CAD build for the part. Positions are in the model's coordinates, mm. A direction names the side the tool comes from. Give positions to 0.01 mm unless a question says otherwise; leave off trailing zeros. Loops run counter-clockwise (first coordinate to the right, second up) from the corner with the lowest first, then second, coordinate; pieces in that order, holes last. Notation, with made-up numbers: M -15,-18.75 L 43,-18.75 A10 cw 43,-0.75 Z; hole C -25.75,65.25 d2. An arc over 180 degrees is marked long. Answer as CSV lines item,"result".
from build123d import *

# Parameters (mm, degrees)
BOSS_EXTRUDE1_DEPTH = 36.83
BOSS_EXTRUDE2_DEPTH = 1.905
SKETCH3_R           = 1.905
CUT_EXTRUDE1_DEPTH  = 2.54
SKETCH4_W           = 7.62
SKETCH4_H           = 3.81
CUT_EXTRUDE2_DEPTH  = 42.576403756


with BuildPart() as part:
    # Sketch1 → Boss-Extrude1 (new body)
    with BuildSketch(Plane(origin=(0, 0, 0), x_dir=(1, 0, 0), z_dir=(0, 1, 0))):
        Polygon((-16.3195, 0), (-6.1595, 0), (-6.1595, 10.287), (0, 10.287), (6.1595, 10.287), (6.1595, 0), (16.3195, 0), (16.3195, 2.54), (8.6995, 2.54), (8.6995, 12.827), (0, 12.827), (-8.6995, 12.827), (-8.6995, 2.54), (-16.3195, 2.54), align=None)
    extrude(amount=-BOSS_EXTRUDE1_DEPTH)

    # Sketch2 → Boss-Extrude2 (add)
    with BuildSketch(Plane(origin=(0, 0, 0), x_dir=(1, 0, 0), z_dir=(0, 1, 0))):
        Polygon((-8.6995, 12.827), (8.6995, 12.827), (8.6995, 0), (3.81, 0), (3.81, 7.62), (-3.81, 7.62), (-3.81, 0), (-8.6995, 0), align=None)
    extrude(amount=-BOSS_EXTRUDE2_DEPTH)

    # Sketch3 → Cut-Extrude1 (cut)
    with BuildSketch(Plane(origin=(0, 0, -2.54), x_dir=(-1, 0, 0), z_dir=(0, 0, -1))):
        with Locations((-12.7, -10.16)):
            Circle(SKETCH3_R)
        with Locations((-12.7, -29.21)):
            Circle(SKETCH3_R)
        with Locations(Location((12.7, -29.21, 0), (0, 0, 180))):
            Circle(SKETCH3_R)
        with Locations(Location((12.7, -10.16, 0), (0, 0, 180))):
            Circle(SKETCH3_R)
    extrude(amount=-CUT_EXTRUDE1_DEPTH, mode=Mode.SUBTRACT)

    # Sketch4 → Cut-Extrude2 (cut, through all)
    with BuildSketch(Plane(origin=(0, 0, -2.54), x_dir=(-1, 0, 0), z_dir=(0, 0, -1))):
        with Locations((-12.5095, -1.905)):
            Rectangle(SKETCH4_W, SKETCH4_H)
        with Locations((12.5095, -1.905)):
            Rectangle(SKETCH4_W, SKETCH4_H)
    extrude(amount=-CUT_EXTRUDE2_DEPTH, mode=Mode.SUBTRACT)


solid = part.part
1) Drill centre lines: line 1 (Y direction, x = 12.7, z = -1.15) (3 decimals); line 2 (X direction, y = -20, z = -4.25); line 3 (Z direction, x = -5.5, y = -9). Where is each one in solid material? Low to high. Write a range as from..to.
Answer below:
line 1,"y = -36.83..-31.115, -27.305..-12.065, -8.255..-3.81"
line 2,"x = -8.7..-6.16, 6.16..8.7"
line 3,"z = -12.83..-10.29"
2) Flat gauge pins, fed straight in: pin 1 (6 mm diameter, centred on y = -14, z = -10.5, fed in from -X); pin 2 (4 mm diameter, centred on x = -11.5, y = -26, fed in from -Z); pin 3 (1 mm diameter, centred on x = -1, y = -1, fed in from +Z); pin 4 (3.5 mm diameter, centred on x = -12.7, y = -29.21, fed in from +Z). Where does each tip first touch, or does it go through?
Answer below:
pin 1,"stops at x = -8.7"
pin 2,"stops at z = -2.54"
pin 3,"stops at z = -7.62"
pin 4,"passes through"
3) Band-saw the part on B-B on y = -10.16. Give the cut face in (x, z) (1 decimal).
Answer below:
outline,"M -16.3,-2.5 L -14.6,-2.5 L -14.6,0 L -16.3,0 Z; M -10.8,-2.5 L -8.7,-2.5 L -8.7,-12.8 L 8.7,-12.8 L 8.7,-2.5 L 10.8,-2.5 L 10.8,0 L 6.2,0 L 6.2,-10.3 L -6.2,-10.3 L -6.2,0 L -10.8,0 Z; M 14.6,-2.5 L 16.3,-2.5 L 16.3,0 L 14.6,0 Z"
4) Mould opens along X. For faces 4 (the face through (0, -19, -10.287)), 5 (the face through (-16.32, -20, -1)), 6 (the face through (-6.16, -19, -5)), 7 (the face through (-12, -20, -2.54)) say: +X half, -X half, draft (parallel to the pull), parting line (faces both ways), or undercut.
Answer below:
face 4,"undercut"
face 5,"-X half"
face 6,"undercut"
face 7,"draft"
5) Band-saw the part on D-D on y = -15. Give the cut face in (x, z).
Answer below:
outline,"M -16.32,-2.54 L -8.7,-2.54 L -8.7,-12.83 L 8.7,-12.83 L 8.7,-2.54 L 16.32,-2.54 L 16.32,0 L 6.16,0 L 6.16,-10.29 L -6.16,-10.29 L -6.16,0 L -16.32,0 Z"
6) Band-saw the part on C-C on x = 12.7. Give the cut face in (y, z) (3 decimals).
Answer below:
outline,"M -36.83,-2.54 L -31.115,-2.54 L -31.115,0 L -36.83,0 Z; M -27.305,-2.54 L -12.065,-2.54 L -12.065,0 L -27.305,0 Z; M -8.255,-2.54 L -3.81,-2.54 L -3.81,0 L -8.255,0 Z"
7) Band-saw the part on A-A on z = -5.75. Give the cut face in (x, y) (1 decimal), and give its area (3 significant figures).
Answer below:
outline,"M -8.7,-36.8 L -6.2,-36.8 L -6.2,-1.9 L -3.8,-1.9 L -3.8,0 L -8.7,0 Z; M 3.8,-1.9 L 6.2,-1.9 L 6.2,-36.8 L 8.7,-36.8 L 8.7,0 L 3.8,0 Z"
area,"196 mm^2"
8) Which spindle directions (+Z, -Z, +X, -X, +Y, -Y) get a long thin tool onto all of the face, cutting with end or side? Do faces 1 (the face through (13, -20, -2.54)), 2 (the face through (3.81, -1, -4)), 3 (the face through (6.16, -19, -5)). Say none if no direction does.
Answer below:
face 1,"-Z, +X, +Y, -Y"
face 2,"+Z, +Y, -Y"
face 3,"+Z, -Y"
